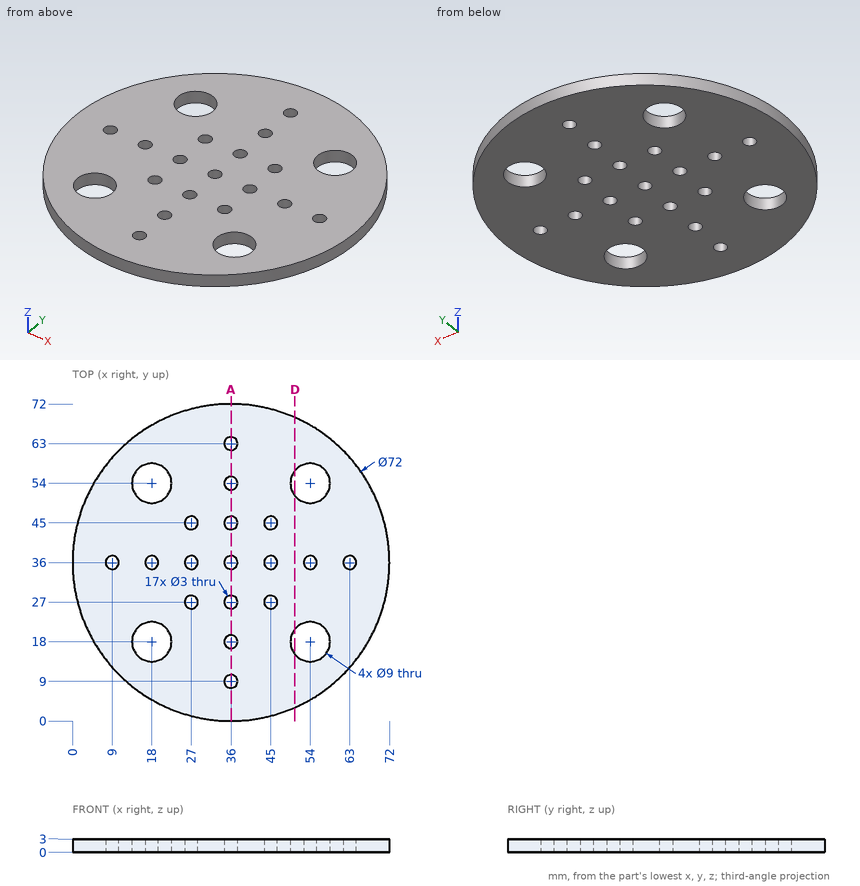
Print and shaded views of the part. All mm, measured from the part's lowest x, y and z. Round coordinates to 2 decimals unless told otherwise and drop trailing zeros. Order: outer loops, then holes, each group sorted by start corner. A loop starts at its lowest first (then second) coordinate and runs counter-clockwise, first axis right, second up. Notation, with made-up numbers: (17, 28) - (70, 28) arc R28 cw to (70, 55) - close; hole circle Ø5 at (9.5, 71.25). An arc over 180 degrees is marked (long way). Use a Markdown table: item, result.
1) Flat gauge pin, fed straight in: pin 1 Ø1 at (y, z) = (47.5, 0.5) entering from -X. Where does the tip first touch, or does it go through?
Recorded:
| item | result |
|---|---|
| pin 1 | stops at x = 1.72 |
2) Saw through at D-D on x = 50.5. Write the cut outline in (y, z), and give its area (3 significant figures).
Recorded:
| item | result |
|---|---|
| outline | (3.05, 0) - (15.17, 0) - (15.17, 3) - (3.05, 3) - close; (20.83, 0) - (51.17, 0) - (51.17, 3) - (20.83, 3) - close; (56.83, 0) - (68.95, 0) - (68.95, 3) - (56.83, 3) - close |
| area | 164 mm² |
3) Saw through at A-A on x = 36. Give the number of separate pieces and of enclosed holes in the cut face, and give its area (3 significant figures).
Recorded:
| item | result |
|---|---|
| separate pieces | 8 |
| enclosed holes | 0 |
| area | 153 mm² |
4) Wall check: L1, parallel to Y at x = 56.5, z = 1.55; L2, parallel to Y at x = 19, z = 1.05; L3, parallel to Y at x = 51, z = 2.8. Give the ranges that are in metal, low to high.
Recorded:
| item | result |
|---|---|
| L1 | y = 6.41 to 14.26, 21.74 to 50.26, 57.74 to 65.59 |
| L2 | y = 4.27 to 13.61, 22.39 to 34.88, 37.12 to 49.61, 58.39 to 67.73 |
| L3 | y = 3.27 to 14.65, 21.35 to 50.65, 57.35 to 68.73 |
